Check sheet for the modelled part. Datum: model origin and axes. Units: mm. A direction names the side the tool comes from. Give positions to 0.01 mm unless a question says otherwise; leave off trailing zeros. Write each loop counter-clockwise with the first axis right and the second up, starting at its lowest first coordinate (ties: lowest second). Pieces come first, ordered by that corner, then holes.
from build123d import *

# Parameters (mm, degrees)
FILLET1_R                = 4
FILLET2_R                = 3
M4_CLEARANCE_HOLE1_D     = 4.5
M4_CLEARANCE_HOLE1_DEPTH = 12
CIRPATTERN1_COUNT        = 3
SKETCH7_W                = 28
SKETCH7_H                = 3
BOSS_EXTRUDE1_DEPTH      = 15


with BuildPart() as part:
    # Sketch2 → Revolve1 (revolve)
    with BuildSketch(Plane.XY):
        with BuildLine():
            Line((0, 8.050125629), (0, -36))
            Line((0, -36), (35, -36))
            Line((35, -36), (35, -20))
            Line((35, -20), (36, -20))
            Line((36, -20), (36, -8))
            Line((36, -8), (35, -8))
            Line((35, -8), (35, -4))
            Line((35, -4), (37, -4))
            Line((37, -4), (37, 0))
            Line((37, 0), (55, 0))
            Line((55, 0), (55, 4))
            Line((55, 4), (17, 4))
            Line((17, 4), (17, 0))
            Line((17, 0), (15, 0))
            ThreePointArc((15, 0), (8.511822993, 5.91041785), (0, 8.050125629))
        make_face()
    revolve(axis=Axis((0, 0, 0), (0, 1, 0)))

    # Fillet1
    fillet1_edges = [part.edges().sort_by_distance(p)[0] for p in [
        (-35, -36, 0),
    ]]
    fillet(fillet1_edges, radius=FILLET1_R)

    # Fillet2
    fillet2_edges = [part.edges().sort_by_distance(p)[0] for p in [
        (-17, 4, 0),
    ]]
    fillet(fillet2_edges, radius=FILLET2_R)

    # M4 Clearance Hole1
    with Locations(Plane(origin=(0, 4, 0), x_dir=(1, 0, 0), z_dir=(0, 1, 0))):
        with Locations((0, 49.5)):
            m4_clearance_hole1 = Hole(M4_CLEARANCE_HOLE1_D / 2, depth=M4_CLEARANCE_HOLE1_DEPTH)

    # Sketch6 → Revolve3 (revolve)
    with BuildSketch(Plane(origin=(0, 0, 0), x_dir=(0, 0, -1), z_dir=(1, 0, 0))):
        with BuildLine():
            Line((33, 4), (30, 4))
            Line((30, 4), (30, 5))
            ThreePointArc((30, 5), (31.58113883, 4.74341649), (33, 4))
        make_face()
    revolve3 = revolve(axis=Axis((0, 5, -30), (0, -1, 0)))

    # CirPattern1: M4 Clearance Hole1, Revolve3 ×3 about axis
    cirpattern1_axis = Axis((0, 0, 0), (0, 1, 0))
    for i in range(1, CIRPATTERN1_COUNT):
        add(m4_clearance_hole1.rotate(cirpattern1_axis, i * 360 / CIRPATTERN1_COUNT), mode=Mode.SUBTRACT)
        add(revolve3.rotate(cirpattern1_axis, i * 360 / CIRPATTERN1_COUNT))

    # Sketch7 → Boss-Extrude1 (add)
    with BuildSketch(Plane.XZ):
        with Locations((0, 41.5)):
            Rectangle(SKETCH7_W, SKETCH7_H)
    extrude(amount=BOSS_EXTRUDE1_DEPTH)


solid = part.part
1) Sectioned sample at B-B on y = -5.5. Record the boundary of the cut face in (x, z), then the cut area to 3 significant figures.
2) Sectioned sample at C-C on z = -49.5. Record the boundary of the cut face in (x, y).
3) Draft check along X on faces 1 (the cylindrical face through (0.29, 1.97, -51.73)), 2 (the cylindrical face through (-11.923, 2.028, 53.692)), 3 (the flat face through (14, -7, 41)), 4 (the flat face through (0, -7, 40)). Enter one of: +X half, -X half, draft (parallel to the pull), parting line (faces both ways), or undercut.
4) Sectioned sample at D-D on y = 2.5. Record the boundary of the cut face in (x, z).
5) Scan lines: L1, parallel to X at y = 2, z = 24; L2, parallel to Z at x = 3, y = 3.5; L3, parallel to Z at x = 0, y = 2. Record each from-to range of solid material in increasing order.
6) Gauge pin test, flat ends, axial feed: pin 1 (10 mm diameter, centred on x = 12, z = -11, fed in from +Y); pin 2 (8 mm diameter, centred on x = 3.5, y = -17.5, fed in from +Z); pin 3 (1.5 mm diameter, centred on y = -6, z = 42, fed in from -X); pin 4 (2.5 mm diameter, centred on x = -42.87, z = 24.75, fed in from -Y). Record the tip position at first contact, or that the pin passes through.
7) Access from +Z, -Z, +X, -X, +Y, -Y to the whole of each face (thin tool, end or side, straight path). Record for faces 5 (the cylindrical face through (9.139, 0.493, -14.334)), 6 (the flat face through (0, -15, 42)), 7 (the flat face through (-14, -7, 41)), 8 (the cylindrical face through (-28, -26, 21)), 9 (the flat face through (-14, -4, 33)).
Answers below:
1. outline: circle Ø70 at (0, 0); (-14, 40) - (14, 40) - (14, 43) - (-14, 43) - close
1. area: 3,930 mm2
2. outline: (-23.97, 0) - (-2.25, 0) - (-2.25, 4) - (-23.97, 4) - close; (2.25, 0) - (23.97, 0) - (23.97, 4) - (2.25, 4) - close
3. face 1: undercut
3. face 2: parting line
3. face 3: +X half
3. face 4: draft
4. outline: circle Ø110 at (0, 0); circle Ø26 at (0, 0); hole circle Ø4.5 at (-42.87, 24.75); hole circle Ø34.8 at (0, 0); hole circle Ø4.5 at (0, -49.5); hole circle Ø4.5 at (42.87, 24.75)
5. L1: x = -49.49 to -44.99, -40.75 to 40.75, 44.99 to 49.49
5. L2: z = -54.92 to -18.09, -11.58 to 11.58, 18.09 to 54.92
5. L3: z = -55 to -51.75, -47.25 to -17.17, -13.46 to 13.46, 17.17 to 55
6. pin 1: stops at y = 4.08
6. pin 2: stops at z = 43
6. pin 3: stops at x = -14
6. pin 4: passes through
7. face 5: +Y
7. face 6: +Z, +X, -X, -Y
7. face 7: +Z, -X, -Y
7. face 8: -Y
7. face 9: none
